Could you check a few things on this model? Use its own coordinates, in mm. A direction names the side the tool comes from. Round coordinates to 2 decimals unless told otherwise and drop trailing zeros. Order: outer loops, then holes, each group sorted by start corner. A loop starts at its lowest first (then second) coordinate and runs counter-clockwise, first axis right, second up. Notation, with made-up numbers: (-28, 61) - (-20, 61) arc R17 ccw to (-20, 77) - close; hole circle Ø6 at (84.5, 10.5). An arc over 180 degrees is marked (long way). Use one line per item in the form item = value.
Autodesk Inventor part; units mm, degrees
ref_plane "YZ Plane" through (0, 0, 0) normal (1, 0, 0) x (0, 1, 0)
ref_plane "XZ Plane" through (0, 0, 0) normal (0, 1, 0) x (-1, 0, 0)
ref_plane "XY Plane" through (0, 0, 0) normal (0, 0, 1) x (1, 0, 0)
sketch "Sketch1" plane through (0, 0, 0) normal (0, 1, 0) x (-1, 0, 0)
  line L0 (232.1908, -176.5808) -> (232.1908, -3.7592)
  arc A0 (232.1908, -3.7592) -> (227.4316, 1) centre (227.4316, -3.7592) ccw
  line L1 (227.4316, 1) -> (0, 1)
  arc A1 (0, 1) -> (-4.7592, -3.7592) centre (0, -3.7592) ccw
  arc A2 (-4.7592, -176.5808) -> (0, -181.34) centre (0, -176.5808) ccw
  arc A3 (227.4316, -181.34) -> (232.1908, -176.5808) centre (227.4316, -176.5808) ccw
  circle A4 centre (130, -129.34) radius 2.25
  circle A5 centre (129.9861, -89.34) radius 2.25
  circle A6 centre (90, -129.34) radius 2.25
  circle A7 centre (89.9861, -89.34) radius 2.25
  circle A8 centre (180, -110) radius 2.75
  circle A9 centre (55, -110) radius 2.75
  circle A10 centre (90, -45) radius 3
  circle A11 centre (190, -45) radius 3
  circle A12 centre (190, -65) radius 3
  circle A13 centre (90, -65) radius 3
  circle A14 centre (140, -45) radius 3
  circle A15 centre (40, -45) radius 3
  circle A16 centre (140, -65) radius 3
  circle A17 centre (40, -65) radius 3
  line L2 (230.1908, -176.5808) -> (230.1908, -3.7592)
  arc A18 (230.1908, -3.7592) -> (227.4316, -1) centre (227.4316, -3.7592) ccw
  line L3 (227.4316, -1) -> (0, -1)
  arc A19 (0, -1) -> (-2.7592, -3.7592) centre (0, -3.7592) ccw
  arc A20 (-2.7592, -176.5808) -> (0, -179.34) centre (0, -176.5808) ccw
  arc A21 (227.4316, -179.34) -> (230.1908, -176.5808) centre (227.4316, -176.5808) ccw
  line L4 (-4.7592, -3.7592) -> (-4.7592, -176.5808)
  line L5 (-2.7592, -3.7592) -> (-2.7592, -176.5808)
  line L6 (0, -179.34) -> (227.4316, -179.34)
  line L7 (227.4316, -181.34) -> (0, -181.34)
  line L8 (0, 0) -> (0, -15)
  line L9 (0, 0) -> (15, 0) construction
  line L10 (0, 0) -> (15, 0)
  line L11 (0, 0) -> (15, 0) construction
  circle A22 centre (20, -155) radius 2.25
  circle A23 centre (76, -155) radius 2.25
  circle A24 centre (20, -99) radius 2.25
  point P0 (230.1908, -3.7592)
  point P1 (0, -1)
  dimension "d0" = 2
  dimension "d1" = 2
  dimension "d2" = 2
  dimension "d3" = 2
  dimension "d5" = 2
  dimension "d7" = 2
  dimension "d8" = 227.4316
  dimension "d9" = 172.8216
  dimension "d10" = 4.7592
  dimension "d45" = 15
  dimension "d46" = 90
  dimension "d47" = 15
  dimension "d48" = 0
  dimension "d49" = 110
  dimension "d50" = 55
  dimension "d51" = 125
  dimension "d52" = 110
  dimension "d54" = 40
  dimension "d55" = 40
  dimension "d56" = 40
  dimension "d57" = 40
  dimension "d58" = 50
  dimension "d59" = 100.1908
  dimension "d60" = 2.7592
  dimension "d61" = 1
  dimension "d62" = 4.7592
  dimension "d63" = 178.34
  dimension "d64" = 180.34
  dimension "d65" = 172.8216
  dimension "d66" = 230.1908
  dimension "d67" = 4.5
  dimension "d68" = 5.5
  dimension "d69" = 6
  dimension "d70" = 40.1908
  dimension "d71" = 64
  dimension "d72" = 20
  dimension "d73" = 50
  dimension "d74" = 50
  dimension "d75" = 50
  dimension "d76" = 20
  dimension "d77" = 20
  dimension "d78" = 20
  dimension "d79" = 50
  dimension "d87" = 4.5
  dimension "d89" = 45
  dimension "d90" = 35
  dimension "d91" = 4.5
  dimension "d92" = 56
  dimension "d93" = 4.5
  dimension "d94" = 56
extrude "Extrusion1" add sketch "Sketch1" along normal blind 6 contours A21 L6 A20 L5 A19 L3 A18 L2
sketch "Sketch2" plane through (0, 6, 0) normal (0, 1, 0) x (1, 0, 0)
  line L0 (-232.1908, 176.5808) -> (-232.1908, 3.7592)
  arc A0 (-232.1908, 3.7592) -> (-227.4316, -1) centre (-227.4316, 3.7592) ccw
  line L1 (-227.4316, -1) -> (0, -1)
  arc A1 (0, -1) -> (4.7592, 3.7592) centre (0, 3.7592) ccw
  arc A2 (4.7592, 176.5808) -> (0, 181.34) centre (0, 176.5808) ccw
  arc A3 (-227.4316, 181.34) -> (-232.1908, 176.5808) centre (-227.4316, 176.5808) ccw
  line L2 (-230.1908, 176.5808) -> (-230.1908, 3.7592)
  arc A4 (-230.1908, 3.7592) -> (-227.4316, 1) centre (-227.4316, 3.7592) ccw
  line L3 (-227.4316, 1) -> (0, 1)
  arc A5 (0, 1) -> (2.7592, 3.7592) centre (0, 3.7592) ccw
  arc A6 (2.7592, 176.5808) -> (0, 179.34) centre (0, 176.5808) ccw
  arc A7 (-227.4316, 179.34) -> (-230.1908, 176.5808) centre (-227.4316, 176.5808) ccw
  line L4 (4.7592, 3.7592) -> (4.7592, 176.5808)
  line L5 (2.7592, 3.7592) -> (2.7592, 176.5808)
  line L6 (0, 179.34) -> (-227.4316, 179.34)
  line L7 (-227.4316, 181.34) -> (0, 181.34)
  line L8 (0, 179.34) -> (-227.4316, 179.34)
  line L9 (-113.7158, 179.34) -> (-113.7158, 1)
  line L10 (-227.4316, 1) -> (0, 1)
  line L11 (-118.7158, 120.17) -> (-108.7158, 120.17)
  line L12 (-108.7158, 120.17) -> (-108.7158, 60.17)
  line L13 (-108.7158, 60.17) -> (-118.7158, 60.17)
  line L14 (-118.7158, 60.17) -> (-118.7158, 120.17)
  line L15 (-118.7158, 120.17) -> (-108.7158, 60.17) construction
  line L16 (-108.7158, 120.17) -> (-118.7158, 60.17) construction
  line L17 (-113.7158, 179.34) -> (-113.7158, 179.34)
  line L18 (2.7592, 159.34) -> (-230.1908, 159.34)
  line L19 (-230.1908, 159.34) -> (-230.1908, 199.34)
  line L20 (-230.1908, 199.34) -> (2.7592, 199.34)
  line L21 (2.7592, 199.34) -> (2.7592, 159.34)
  line L22 (2.7592, 159.34) -> (-230.1908, 199.34) construction
  line L23 (-230.1908, 159.34) -> (2.7592, 199.34) construction
  line L24 (-113.7158, 1) -> (-113.7158, 16)
  line L25 (-230.1908, 31) -> (2.7592, 31)
  line L26 (2.7592, 31) -> (2.7592, 1)
  line L27 (2.7592, 1) -> (-230.1908, 1)
  line L28 (-230.1908, 1) -> (-230.1908, 31)
  line L29 (-230.1908, 31) -> (2.7592, 1) construction
  line L30 (2.7592, 31) -> (-230.1908, 1) construction
  line L31 (-227.4316, 1) -> (0, 1)
  line L32 (-230.1908, 199.34) -> (-200.1908, 199.34)
  line L33 (-200.1908, 199.34) -> (-200.1908, 1)
  line L34 (-200.1908, 1) -> (-230.1908, 1)
  line L35 (-230.1908, 1) -> (-230.1908, 199.34)
  line L36 (2.7592, 1) -> (-7.2408, 1)
  line L37 (-7.2408, 1) -> (-7.2408, 199.34)
  line L38 (-7.2408, 199.34) -> (2.7592, 199.34)
  line L39 (2.7592, 199.34) -> (2.7592, 1)
  point P0 (230.1908, -176.5808)
  point P1 (230.1908, -3.7592)
  point P2 (227.4316, -1)
  point P3 (0, -1)
  point P4 (0, 0)
  point P5 (230.1908, -176.5808)
  point P6 (230.1908, -3.7592)
  point P7 (227.4316, -1)
  point P8 (0, -1)
  point P9 (-113.7158, 90.17)
  point P10 (-113.7158, 120.17)
  point P11 (-113.7158, 60.17)
  point P12 (-113.7158, 1)
  point P13 (0, 1)
  point P14 (-230.1908, 3.7592)
  point P15 (-227.4316, 1)
  point P16 (-113.7158, 159.34)
  point P17 (-7.2408, 159.34)
  point P18 (-7.2408, 31)
  point P19 (-113.7158, 31)
  point P20 (2.7592, 3.7592)
  point P21 (2.7592, 176.5808)
  point P22 (-7.2408, 179.34)
  point P23 (-200.1908, 159.34)
  point P24 (-200.1908, 31)
  dimension "d22" = 2
  dimension "d23" = 2
  dimension "d24" = 2
  dimension "d25" = 2
  dimension "d26" = 2
  dimension "d27" = 2
  dimension "d28" = 227.4316
  dimension "d29" = 172.8216
  dimension "d30" = 4.7592
  dimension "d31" = 10
  dimension "d32" = 60
  dimension "d37" = 0
  dimension "d38" = 40
  dimension "d39" = 15
  dimension "d40" = 30
  dimension "d41" = 30
  dimension "d42" = 10
extrude "Extrusion4" cut sketch "Sketch2" against normal through all contours A7 L6 L33 L18 L2 | L18 L33 L25 L2 | L37 L20 L21 A2 L7 | L7 A2 L21 A6 L6 L37 | L6 L9 L18 L33 | L25 L33 L3 A4 L2 | L37 L18 L9 L6 | L6 A6 L5 L18 L37 | L25 L9 L3 L33 | L18 L37 L25 L9 L13 L12 L11 | L18 L5 L25 L37 | L25 L37 L3 L9 | L11 L12 L13 L9 | L9 L13 L14 L11 | L25 L5 A5 L3 L37 | L26 L27 A5
fillet "Fillet4" radius 2 6 edges at (-113.7158, 3, -31) (-200.1908, 3, -31) (-118.7158, 3, -120.17) (-118.7158, 3, -60.17) (-113.7158, 3, -159.34) (-200.1908, 3, -159.34)
equation "\"d1\" = d0"
equation "\"d2\" = d0"
equation "\"d3\" = d0"
equation "\"d5\" = d0"
equation "\"d7\" = d0"
equation "\"d23\" = d22"
equation "\"d24\" = d22"
equation "\"d25\" = d22"
equation "\"d26\" = d22"
equation "\"d27\" = d22"
properties part number "EboxBottom_1"
Item 1: Imagine slicing it at C-C on x = -180. Please give me the cut outline in (y, z).
Found:
outline = (0, -159.34) - (6, -159.34) - (6, -112.75) - (0, -112.75) - close; (0, -107.25) - (6, -107.25) - (6, -31) - (0, -31) - close
Item 2: Imagine slicing it at B-B on z = -89.34. Please give me the cut outline in (x, y), plus the area to 3 significant figures.
Found:
outline = (-200.19, 0) - (-132.24, 0) - (-132.24, 6) - (-200.19, 6) - close; (-127.74, 0) - (-118.72, 0) - (-118.72, 6) - (-127.74, 6) - close
area = 462 mm2
Item 3: Will this pin go through, and if not, where does the flat tip stop? P1, Ø5.5, axis at x = -190, z = -65, coming from the -Y side.
Found:
P1 = through
Item 4: Imagine slicing it at D-D on z = -65. Please give me the cut outline in (x, y).
Found:
outline = (-200.19, 0) - (-193, 0) - (-193, 6) - (-200.19, 6) - close; (-187, 0) - (-143, 0) - (-143, 6) - (-187, 6) - close; (-137, 0) - (-118.72, 0) - (-118.72, 6) - (-137, 6) - close
Item 5: If we mould it in two halves opening along Z, with no side actions, what happens to faces 1 (the face through (-156, 3, -159.34)), 2 (the face through (-115, 3, -60.17)), 3 (the face through (-142.86, 2.96, -45.9)), 4 (the face through (-156, 0, -94))? For each: released by +Z, released by -Z, zero draft, split by the parting line, or undercut.
Found:
face_1 = released by -Z
face_2 = undercut
face_3 = undercut
face_4 = zero draft
Item 6: Imagine slicing it at A-A on x = -190. Please give me the cut outline in (y, z).
Found:
outline = (0, -159.34) - (6, -159.34) - (6, -68) - (0, -68) - close; (0, -62) - (6, -62) - (6, -48) - (0, -48) - close; (0, -42) - (6, -42) - (6, -31) - (0, -31) - close
Item 7: For faces 5 (the face through (-115, 3, -120.17)), 6 (the face through (-191.384, 2.958, -62.338)), which set-ups out of +Z, -Z, +X, -X, +Y, -Y let a thin tool reach every point of the face, with its end or its side?
Found:
face_5 = +X, +Y, -Y
face_6 = +Y, -Y
Item 8: I need wall thicknesses on L1, parallel to Z at x = -140, y = 2.65; L2, parallel to Z at x = -180, y = 4.65; L3, parallel to X at y = 4.15, z = -129.34. Which ranges of each line are inside material? Lowest first, please.
Found:
L1 = -159.34 to -68, -62 to -48, -42 to -31
L2 = -159.34 to -112.75, -107.25 to -31
L3 = -200.19 to -132.25, -127.75 to -113.72
